Source: three-view drawing plus pictorial views. Frame: mm from the lowest corner of the part. A direction names the side the tool comes from. Give positions to 0.01 mm unless a question says otherwise; leave off trailing zeros. Loops run counter-clockwise (first coordinate to the right, second up) from the corner with the lowest first, then second, coordinate; pieces in that order, holes last.
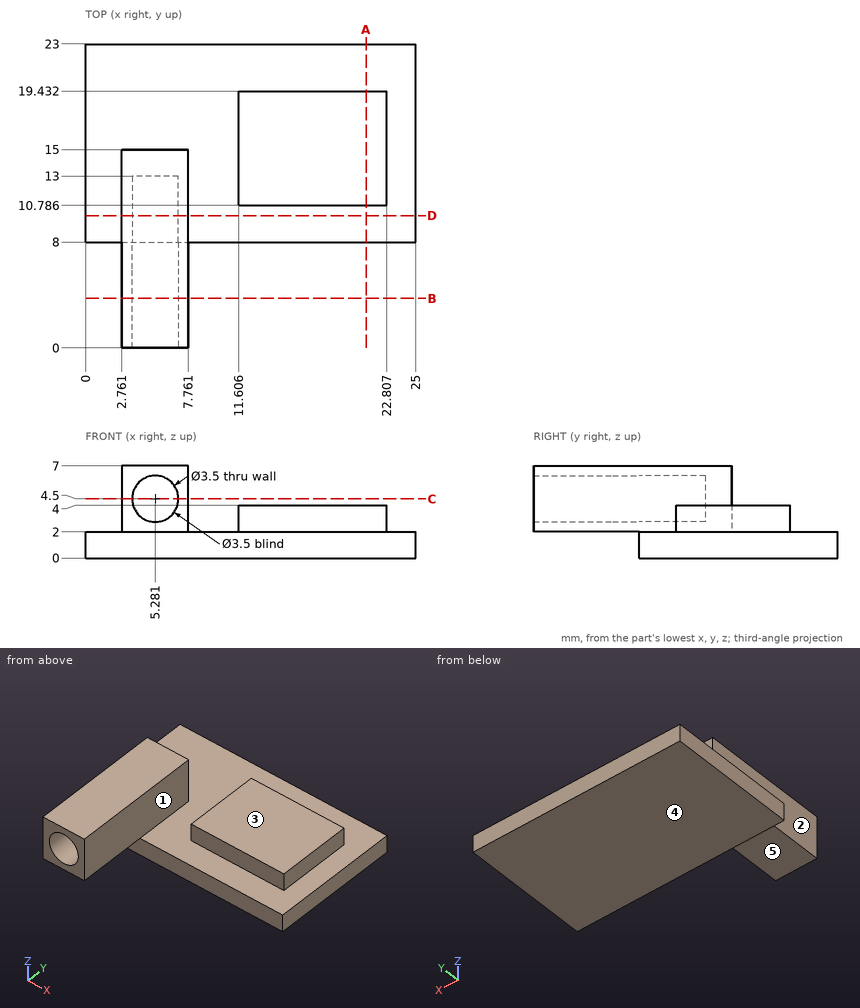
1) Cut plane A-A (x = 21.25). Return loops of the section in (y, z).
Checks:
outline: (8, 0) - (23, 0) - (23, 2) - (19.43, 2) - (19.43, 4) - (10.79, 4) - (10.79, 2) - (8, 2) - close
2) Contact query for flat-ended pins moving along their axis: P1, Ø1.5, axis at y = 15, z = 6, coming from the -X side; P2, Ø1, axis at x = 18, z = 3, coming from the +Y side; P3, Ø3, axis at x = 5.28, z = 4.5, coming from the +Y side. Output: stop coordinate, or through.
Checks:
P1: stops at x = 2.76
P2: stops at y = 19.43
P3: stops at y = 15
3) Cut plane C-C (z = 4.5). Return loops of the section in (x, y).
Checks:
outline: (2.76, 0) - (3.53, 0) - (3.53, 13) - (7.03, 13) - (7.03, 0) - (7.76, 0) - (7.76, 15) - (2.76, 15) - close
4) Cut plane B-B (y = 3.75). Return loops of the section in (x, z), and give its area (3 significant figures).
Checks:
outline: (2.76, 2) - (7.76, 2) - (7.76, 7) - (2.76, 7) - close; hole circle Ø3.5 at (5.28, 4.5)
area: 15.4 mm2
5) Cut plane D-D (y = 10). Return loops of the section in (x, z).
Checks:
outline: (0, 0) - (25, 0) - (25, 2) - (7.76, 2) - (7.76, 7) - (2.76, 7) - (2.76, 2) - (0, 2) - close; hole circle Ø3.5 at (5.28, 4.5)
6) Ray query, probe 1 along Y at (x, z) = (16.75, 2.75); probe 2 along Y at (x, z) = (19.5, 1.75); probe 3 along Z at (x, y) = (14.5, 21.5). Return the intervals inside material, ascending.
Checks:
probe 1: y = 10.79 to 19.43
probe 2: y = 8 to 23
probe 3: z = 0 to 2
7) Reachability of the marked faces 1, 2, 3, 4 and 5 from +Z, -Z, +X, -X, +Y, -Y: full face, straight path, thin tool, end or side. Return the list, or none.
Checks:
face 1: +Z, +Y, -Y
face 2: +Z, -X, +Y, -Y
face 3: +Z, +X, +Y, -Y
face 4: -Z, +X, -X, +Y, -Y
face 5: -Z, +X, -X, -Y
